```python
from build123d import *

# Parameters (mm, degrees)
SKETCH_2_W          = 180
SKETCH_2_H          = 180
EXTRUDE_1_DEPTH     = 3
SKETCH_3_R          = 4.1
CUT_EXTRUDE_1_DEPTH = 3
SKETCH_4_OUTSIDE_W  = 232.916
SKETCH_4_OUTSIDE_H  = 232.916
SKETCH_4_OUTSIDE_R  = 100
CUT_EXTRUDE_2_DEPTH = 3
SKETCH_5_R          = 1.55
CUT_EXTRUDE_3_DEPTH = 3
FILLET_1_R          = 2
SKETCH_7_R          = 22.5
CUT_EXTRUDE_4_DEPTH = 10
CUT_EXTRUDE_5_DEPTH = 10
FILLET_2_R          = 10
CHAMFER_1_SIZE      = 1.5
CHAMFER_1_SIZE2     = 2.598076211


with BuildPart() as part:
    # 草图2 → 凸台-拉伸1 (new body)
    with BuildSketch(Plane(origin=(0, 0, 0), x_dir=(1, 0, 0), z_dir=(0, 1, 0))):
        Rectangle(SKETCH_2_W, SKETCH_2_H)
    extrude(amount=EXTRUDE_1_DEPTH)

    # 草图3 → 切除-拉伸1 (cut)
    with BuildSketch(Plane(origin=(0, 3, 0), x_dir=(1, 0, 0), z_dir=(0, 1, 0))):
        with Locations(Location((0, 40, 0), (0, 0, 270))):
            Circle(SKETCH_3_R)
        with Locations(Location((28.284271247, 28.284271247, 0), (0, 0, 270))):
            Circle(SKETCH_3_R)
        with Locations(Location((40, 0, 0), (0, 0, 270))):
            Circle(SKETCH_3_R)
        with Locations(Location((28.284271247, -28.284271247, 0), (0, 0, 270))):
            Circle(SKETCH_3_R)
        with Locations(Location((0, -40, 0), (0, 0, 270))):
            Circle(SKETCH_3_R)
        with Locations(Location((-28.284271247, -28.284271247, 0), (0, 0, 270))):
            Circle(SKETCH_3_R)
        with Locations(Location((-40, 0, 0), (0, 0, 270))):
            Circle(SKETCH_3_R)
        with Locations(Location((-28.284271247, 28.284271247, 0), (0, 0, 270))):
            Circle(SKETCH_3_R)
    extrude(amount=-CUT_EXTRUDE_1_DEPTH, mode=Mode.SUBTRACT)

    # 草图4 outside → 切除-拉伸2 (cut)
    with BuildSketch(Plane(origin=(0, 3, 0), x_dir=(1, 0, 0), z_dir=(0, 1, 0))):
        Rectangle(SKETCH_4_OUTSIDE_W, SKETCH_4_OUTSIDE_H)
        Circle(SKETCH_4_OUTSIDE_R, mode=Mode.SUBTRACT)
    extrude(amount=-CUT_EXTRUDE_2_DEPTH, mode=Mode.SUBTRACT)

    # 草图5 → 切除-拉伸3 (cut)
    with BuildSketch(Plane(origin=(0, 3, 0), x_dir=(1, 0, 0), z_dir=(0, 1, 0))):
        with Locations(Location((-85, 8, 0), (0, 0, 270))):
            Circle(SKETCH_5_R)
        with Locations(Location((-70, 8, 0), (0, 0, 270))):
            Circle(SKETCH_5_R)
        with Locations(Location((-85, -8, 0), (0, 0, 270))):
            Circle(SKETCH_5_R)
        with Locations(Location((-70, -8, 0), (0, 0, 270))):
            Circle(SKETCH_5_R)
        with Locations(Location((70, -8, 0), (0, 0, 90))):
            Circle(SKETCH_5_R)
        with Locations(Location((85, -8, 0), (0, 0, 90))):
            Circle(SKETCH_5_R)
        with Locations(Location((70, 8, 0), (0, 0, 90))):
            Circle(SKETCH_5_R)
        with Locations(Location((85, 8, 0), (0, 0, 90))):
            Circle(SKETCH_5_R)
    extrude(amount=-CUT_EXTRUDE_3_DEPTH, mode=Mode.SUBTRACT)

    # 圆角1
    fillet_1_edges = [part.edges().sort_by_distance(p)[0] for p in [
        (-90, 1.5, -43.588989435),
        (-90, 1.5, 43.588989435),
        (-43.588989435, 1.5, 90),
        (43.588989435, 1.5, 90),
        (90, 1.5, 43.588989435),
        (90, 1.5, -43.588989435),
        (43.588989435, 1.5, -90),
        (-43.588989435, 1.5, -90),
    ]]
    fillet(fillet_1_edges, radius=FILLET_1_R)

    # 草图7 → 切除-拉伸4 (cut)
    with BuildSketch(Plane(origin=(0, 3, 0), x_dir=(1, 0, 0), z_dir=(0, 1, 0))):
        with Locations(Location((0, 0, 0), (0, 0, 270))):
            Circle(SKETCH_7_R)
    extrude(amount=-CUT_EXTRUDE_4_DEPTH, mode=Mode.SUBTRACT)

    # 草图8 → 切除-拉伸5 (cut)
    with BuildSketch(Plane(origin=(0, 3, 0), x_dir=(1, 0, 0), z_dir=(0, 1, 0))):
        with BuildLine():
            ThreePointArc((44.007874802, 89.795918367), (43.579471257, 89.948311671), (43.127717306, 90))
            Line((43.127717306, 90), (-43.127717306, 90))
            ThreePointArc((-43.127717306, 90), (-43.579471257, 89.948311671), (-44.007874802, 89.795918367))
            ThreePointArc((-44.007874802, 89.795918367), (-65.640873182, 75.440544589), (-82.849260709, 56))
            ThreePointArc((-82.849260709, 56), (0, 80), (82.849260709, 56))
            ThreePointArc((82.849260709, 56), (65.640873182, 75.440544589), (44.007874802, 89.795918367))
        make_face()
        with BuildLine():
            ThreePointArc((-44.007874802, -89.795918367), (-43.579471257, -89.948311671), (-43.127717306, -90))
            Line((-43.127717306, -90), (43.127717306, -90))
            ThreePointArc((43.127717306, -90), (43.579471257, -89.948311671), (44.007874802, -89.795918367))
            ThreePointArc((44.007874802, -89.795918367), (65.640873182, -75.440544589), (82.849260709, -56))
            ThreePointArc((82.849260709, -56), (0, -80), (-82.849260709, -56))
            ThreePointArc((-82.849260709, -56), (-65.640873182, -75.440544589), (-44.007874802, -89.795918367))
        make_face()
    extrude(amount=-CUT_EXTRUDE_5_DEPTH, mode=Mode.SUBTRACT)

    # 圆角2
    fillet_2_edges = [part.edges().sort_by_distance(p)[0] for p in [
        (82.849260709, 1.5, -56),
        (-82.849260709, 1.5, -56),
        (-82.849260709, 1.5, 56),
        (82.849260709, 1.5, 56),
    ]]
    fillet(fillet_2_edges, radius=FILLET_2_R)

    # 倒角1
    chamfer_1_edges = [part.edges().sort_by_distance(p)[0] for p in [
        (70, 3, 9.55),
        (-70, 3, 6.45),
        (-85, 3, 6.45),
        (-70, 3, -9.55),
        (85, 3, -6.45),
        (70, 3, -6.45),
        (85, 3, 9.55),
        (-85, 3, -9.55),
    ]]
    chamfer_1_side = [part.faces().sort_by_distance(p)[0] for p in [
        (-85.005243711, 3, -47.940012077),
    ]]
    chamfer(chamfer_1_edges, length=CHAMFER_1_SIZE, length2=CHAMFER_1_SIZE2, reference=chamfer_1_side[0])


solid = part.part
```
Can you work these out from the model? Positions are in its coordinate system, mm. Round coordinates to 2 decimals unless told otherwise and drop trailing zeros. Loops run counter-clockwise (first coordinate to the right, second up) from the corner with the lowest first, then second, coordinate; pieces in that order, holes last.
Item 1: Suppose I cut it at D-D, the plane x = -40. Write out the boundary of the cut face in (y, z), then the cut area to 3 significant figures.
Item 2: Suppose I cut it at B-B, the plane x = 0. Write out the boundary of the cut face in (y, z).
Item 3: If we mould it in two halves opening along Z, with no side actions, what happens to faces 1 (the cylindrical face through (-1.192, 1.521, -79.995)), 2 (the flat face through (19, 0, 17)), 3 (the cylindrical face through (32.35, 1.52, -28.82)), 4 (the conical face through (86.75, 0.82, -7.61))? For each: +Z half, -Z half, draft (parallel to the pull), parting line (faces both ways), or undercut.
Item 4: Suppose I cut it at C-C, the plane z = 0. Write out the boundary of the cut face in (x, y), then the cut area to 3 significant figures.
Item 5: Will these pins go through, and if not, where does the flat tip stop? pin 1 Ø6.5 at (x, z) = (-28.28, 28.28) entering from +Y; pin 2 Ø5 at (x, z) = (85, 8) entering from +Y.
Item 6: Suppose I cut it at A-A, the plane z = -40. Write out the boundary of the cut face in (x, y).
Item 7: Please list where these lines run through material, in increasing order: L1, parallel to X at y = 0.6, z = 0; L2, parallel to X at y = 0.6, z = 40; L3, parallel to Z at x = 70.5, y = 1.05.
Reported:
1. outline: (0, -74.75) - (3, -74.75) - (3, -4.1) - (0, -4.1) - close; (0, 4.1) - (3, 4.1) - (3, 74.75) - (0, 74.75) - close
1. area: 424 mm2
2. outline: (0, -80) - (3, -80) - (3, -44.1) - (0, -44.1) - close; (0, -35.9) - (3, -35.9) - (3, -22.5) - (0, -22.5) - close; (0, 22.5) - (3, 22.5) - (3, 35.9) - (0, 35.9) - close; (0, 44.1) - (3, 44.1) - (3, 80) - (0, 80) - close
3. face 1: -Z half
3. face 2: draft
3. face 3: undercut
3. face 4: undercut
4. outline: (-90, 0) - (-44.1, 0) - (-44.1, 3) - (-90, 3) - close; (-35.9, 0) - (-22.5, 0) - (-22.5, 3) - (-35.9, 3) - close; (22.5, 0) - (35.9, 0) - (35.9, 3) - (22.5, 3) - close; (44.1, 0) - (90, 0) - (90, 3) - (44.1, 3) - close
4. area: 356 mm2
5. pin 1: passes through
5. pin 2: stops at y = 2.05
6. outline: (-90, 0) - (-4.1, 0) - (-4.1, 3) - (-90, 3) - close; (4.1, 0) - (90, 0) - (90, 3) - (4.1, 3) - close
7. L1: x = -90 to -44.1, -35.9 to -22.5, 22.5 to 35.9, 44.1 to 90
7. L2: x = -90 to -4.1, 4.1 to 90
7. L3: z = -63.04 to -9.86, -6.14 to 6.14, 9.86 to 63.04
